Work out the finished part from the listing and answer in its coordinate system (mm). Round coordinates to 2 decimals unless told otherwise and drop trailing zeros. Order: outer loops, then holes, each group sorted by start corner. A loop starts at its lowest first (then second) coordinate and runs counter-clockwise, first axis right, second up. Notation, with made-up numbers: (-8.5, 80.25) -> (23.5, 80.25) arc R19 cw to (23.5, 107.25) -> close; hole circle Ø11 at (1.5, 48). An arc over 180 degrees is marked (long way). Use a Markdown table: item, result. Add a question column.
Item 1: A cutting plane is placed at C-C, the plane x = 21.5. Determine the outline of the cut face in (y, z).
Item 2: A cutting plane is placed at B-B, the plane x = 9. Determine the outline of the cut face in (y, z).
Item 3: For a pull along Z with two mould halves and no side action, classify faces 1 (the cylindrical face through (10.62, -0.3, -0.07)), 2 (the flat face through (0, 0, 0)), 3 (the conical face through (0.174, -3.147, -0.413)) as +Z half, -Z half, draft (parallel to the pull), parting line (faces both ways), or undercut.
Item 4: A cutting plane is placed at A-A, the plane y = 0. Determine the outline of the cut face in (x, z), plus the area to 3 significant figures.
Item 5: Flat-ended cylindrical pins translate along their axes: P1, Ø3, axis at x = 52.5, z = 2.5, coming from the -Y side; P2, Ø1.5, axis at y = -1.5, z = 2.5, coming from the -X side. Find the tip coordinate at first contact, or state that the pin passes through.
Item 6: Find the intervals of material crossed by L1, parallel to Z at x = 9, y = -1.75; L2, parallel to Y at x = 43, z = -3.5; L3, parallel to X at y = -0.25, z = 1, in increasing order. Write a range as [from, to].
from build123d import *

# Parameters (mm, degrees)
SKETCH1_W          = 60
SKETCH1_H          = 4
CHAMFER1_SIZE      = 1
CUT_EXTRUDE1_DEPTH = 61.266076693
TAP1_D             = 3.242


with BuildPart() as part:
    # Sketch1 → Revolve1 (revolve)
    with BuildSketch(Plane.XY, mode=Mode.PRIVATE) as revolve1_sk:
        with Locations((30, 2)):
            Rectangle(SKETCH1_W, SKETCH1_H)
    revolve(revolve1_sk.sketch.rotate(Axis((0, 0, 0), (1, 0, 0)), 90), axis=Axis((0, 0, 0), (1, 0, 0)))

    # Chamfer1
    chamfer1_edges = [part.edges().sort_by_distance(p)[0] for p in [
        (60, 0, -4),
        (0, 0, -4),
    ]]
    chamfer(chamfer1_edges, length=CHAMFER1_SIZE)

    # Sketch2 → Cut-Extrude1 (cut, through all)
    with BuildSketch(Plane(origin=(0, 0, 0), x_dir=(0, 0, -1), z_dir=(1, 0, 0))):
        with BuildLine():
            Line((-1.936491673, 3.5), (1.936491673, 3.5))
            ThreePointArc((1.936491673, 3.5), (0, 4), (-1.936491673, 3.5))
        make_face()
    extrude(amount=CUT_EXTRUDE1_DEPTH, mode=Mode.SUBTRACT)

    # Tap1 (through all)
    with Locations(Plane(origin=(0, 3.5, 0), x_dir=(1, 0, 0), z_dir=(0, 1, 0))):
        with Locations((9, 0)):
            Hole(TAP1_D / 2)


solid = part.part
Reported:
| question | item | result |
|---|---|---|
| 1 | outline | (3.5, -1.94) -> (3.5, 1.94) arc R4 ccw (long way) to start |
| 2 | outline | (-3.66, -1.62) arc R4 ccw to (3.5, -1.94) -> (3.5, -1.62) -> close; (-3.66, 1.62) -> (3.5, 1.62) -> (3.5, 1.94) arc R4 ccw to start |
| 3 | face 1 | undercut |
| 3 | face 2 | draft |
| 3 | face 3 | parting line |
| 4 | outline | (0, -3) -> (1, -4) -> (59, -4) -> (60, -3) -> (60, 3) -> (59, 4) -> (1, 4) -> (0, 3) -> close; hole circle Ø3.24 at (9, 0) |
| 4 | area | 470 mm² |
| 5 | P1 | y = -3.87 |
| 5 | P2 | x = 0 |
| 6 | L1 | [-3.6, -1.62], [1.62, 3.6] |
| 6 | L2 | [-1.94, 1.94] |
| 6 | L3 | [0, 7.72], [10.28, 60] |
